Part model, mm, in its own coordinate system. A direction names the side the tool comes from. Coordinates: 2 decimals unless noted, no trailing zeros. Write each loop counter-clockwise with the first axis right and the second up, starting at its lowest first coordinate (ties: lowest second). Pieces come first, ordered by that corner, then holes. Notation, with made-up numbers: M 5.25,8.5 L 9.25,8.5 A11 cw 9.25,12.5 Z; hole C -12,-3 d7. An arc over 180 degrees is marked long. Use a Markdown table: item, result. Add a question column.
Q1. Slice it at A-A on y = 5. Write the cut outline in (x, z), then the cut area to 3 significant figures.
Q2. Wall check: L1, parallel to Z at x = 65, y = 20; L2, parallel to Z at x = 3.75, y = 5; L3, parallel to X at y = 31, z = 45.5. Give the ranges that are in metal, low to high. Write a range as from..to.
Q3. Slice it at B-B on z = 27.5. Write the cut outline in (x, y), then the cut area to 3 significant figures.
Q4. Mould opens along Y. For faces 6 (the cylindrical face through (3.451, 23.845, 6.021)), 7 (the flat face through (35, 46, 90)), 8 (the flat face through (35, 55, 44)) say: released by +Y, released by -Y, zero draft, split by the parting line, or undercut.
Q5. Tool access for faces 1 (the flat face through (35, 45, 44)), 2 (the flat face through (3, 0, 44)), 3 (the flat face through (35, 46, 0)), 4 (the cylindrical face through (3.45, 25.16, 49.74)), 5 (the cylindrical face through (66.55, 39.73, 61.11)): list every direction of +Z, -Z, +X, -X, +Y, -Y with a clear straight run to the whole face (end or side of a thin tool).
Q6. Slice it at D-D on y = 11. Write the cut outline in (x, z).
Q7. Slice it at C-C on y = 40. Write the cut outline in (x, z).
Q8. Pin check, flat tips, straight feed: pin 1 Ø1.5 at (y, z) = (20, 33.33) entering from +X; pin 2 Ø2 at (y, z) = (5, 77.5) entering from -X; pin 3 Ø4 at (y, z) = (5, 14.5) entering from -X; pin 4 Ø5.5 at (x, z) = (66, 33.5) entering from -Y. Stop position of each tip, or through.
from build123d import *

# Parameters (mm, degrees)
SKETCH1_W               = 70
SKETCH1_H               = 55
BOSS_EXTRUDE1_DEPTH     = 90
CUT_EXTRUDE1_DEPTH      = 127.589889012
CUT_EXTRUDE1_DEPTH_BACK = 127.589889012
SKETCH3_R               = 1.25
CUT_EXTRUDE2_DEPTH      = 7
SKETCH4_R               = 1.25
CUT_EXTRUDE4_DEPTH      = 7


with BuildPart() as part:
    # Sketch1 → Boss-Extrude1 (new body)
    with BuildSketch(Plane.XY):
        with Locations((35, 27.5)):
            Rectangle(SKETCH1_W, SKETCH1_H)
    extrude(amount=BOSS_EXTRUDE1_DEPTH)

    # Sketch2 → Cut-Extrude1 (cut, two sides: drawn at the far end of the back side and taken through both)
    with BuildSketch(Plane.XY.offset(90).offset(-CUT_EXTRUDE1_DEPTH_BACK)):
        Polygon((7, 0), (7, 45), (63, 45), (63, 15), (70, 15), (70, 0), (60, 0), align=None)
    extrude(amount=CUT_EXTRUDE1_DEPTH + CUT_EXTRUDE1_DEPTH_BACK, mode=Mode.SUBTRACT)

    # Sketch3 → Cut-Extrude2 (cut)
    with BuildSketch(Plane.ZY):
        with Locations(Location((6.5, 25, 0), (0, 0, 270))):
            Circle(SKETCH3_R)
        with Locations(Location((14.5, 5, 0), (0, 0, 270))):
            Circle(SKETCH3_R)
        with Locations(Location((27.5, 25, 0), (0, 0, 270))):
            Circle(SKETCH3_R)
        with Locations(Location((35.5, 5, 0), (0, 0, 270))):
            Circle(SKETCH3_R)
        with Locations(Location((48.5, 25, 0), (0, 0, 270))):
            Circle(SKETCH3_R)
        with Locations(Location((56.5, 5, 0), (0, 0, 270))):
            Circle(SKETCH3_R)
        with Locations(Location((69.5, 25, 0), (0, 0, 270))):
            Circle(SKETCH3_R)
        with Locations(Location((77.5, 5, 0), (0, 0, 270))):
            Circle(SKETCH3_R)
    extrude(amount=-CUT_EXTRUDE2_DEPTH, mode=Mode.SUBTRACT)

    # Sketch4 → Cut-Extrude4 (cut)
    with BuildSketch(Plane(origin=(70, 0, 0), x_dir=(0, 0, -1), z_dir=(1, 0, 0))):
        with Locations(Location((-83.331764561, 40, 0), (0, 0, 90))):
            Circle(SKETCH4_R)
        with Locations(Location((-75.331764561, 20, 0), (0, 0, 90))):
            Circle(SKETCH4_R)
        with Locations(Location((-62.331764561, 40, 0), (0, 0, 90))):
            Circle(SKETCH4_R)
        with Locations(Location((-54.331764561, 20, 0), (0, 0, 90))):
            Circle(SKETCH4_R)
        with Locations(Location((-41.331764561, 40, 0), (0, 0, 90))):
            Circle(SKETCH4_R)
        with Locations(Location((-33.331764561, 20, 0), (0, 0, 90))):
            Circle(SKETCH4_R)
        with Locations(Location((-20.331764561, 40, 0), (0, 0, 90))):
            Circle(SKETCH4_R)
        with Locations(Location((-12.331764561, 20, 0), (0, 0, 90))):
            Circle(SKETCH4_R)
    extrude(amount=-CUT_EXTRUDE4_DEPTH, mode=Mode.SUBTRACT)


solid = part.part
Recorded:
| question | item | result |
|---|---|---|
| 1 | outline | M 0,0 L 7,0 L 7,13.25 L 0,13.25 Z; M 0,15.75 L 7,15.75 L 7,34.25 L 0,34.25 Z; M 0,36.75 L 7,36.75 L 7,55.25 L 0,55.25 Z; M 0,57.75 L 7,57.75 L 7,76.25 L 0,76.25 Z; M 0,78.75 L 7,78.75 L 7,90 L 0,90 Z |
| 1 | area | 560 mm² |
| 2 | L1 | 0..11.08, 13.58..32.08, 34.58..53.08, 55.58..74.08, 76.58..90 |
| 2 | L2 | 0..13.25, 15.75..34.25, 36.75..55.25, 57.75..76.25, 78.75..90 |
| 2 | L3 | 0..7, 63..70 |
| 3 | outline | M 0,0 L 7,0 L 7,23.75 L 0,23.75 Z; M 0,26.25 L 7,26.25 L 7,45 L 63,45 L 63,15 L 70,15 L 70,55 L 0,55 Z |
| 3 | area | 1,210 mm² |
| 4 | face 6 | undercut |
| 4 | face 7 | zero draft |
| 4 | face 8 | released by +Y |
| 5 | face 1 | +Z, -Z, -Y |
| 5 | face 2 | +Z, -Z, +X, -X, -Y |
| 5 | face 3 | -Z, +X, -X, +Y, -Y |
| 5 | face 4 | -X |
| 5 | face 5 | +X |
| 6 | outline | M 0,0 L 7,0 L 7,90 L 0,90 Z |
| 7 | outline | M 0,0 L 7,0 L 7,90 L 0,90 Z; M 63,0 L 70,0 L 70,19.08 L 63,19.08 Z; M 63,21.58 L 70,21.58 L 70,40.08 L 63,40.08 Z; M 63,42.58 L 70,42.58 L 70,61.08 L 63,61.08 Z; M 63,63.58 L 70,63.58 L 70,82.08 L 63,82.08 Z; M 63,84.58 L 70,84.58 L 70,90 L 63,90 Z |
| 8 | pin 1 | x = 7 |
| 8 | pin 2 | through |
| 8 | pin 3 | x = 0 |
| 8 | pin 4 | y = 15 |
